Part print with two shaded views. Sizes in mm from the minimum x, y, z corner. Round coordinates to 2 decimals unless told otherwise and drop trailing zeros. Order: outer loops, then holes, each group sorted by start corner. A loop starts at its lowest first (then second) coordinate and runs counter-clockwise, first axis right, second up. Notation, with made-up numbers: (26, -2) - (80, -2) arc R20 cw to (80, 13) - close; hole circle Ø7 at (86.5, 31.5). An arc over 180 degrees is marked (long way). Write item = value, one per line.
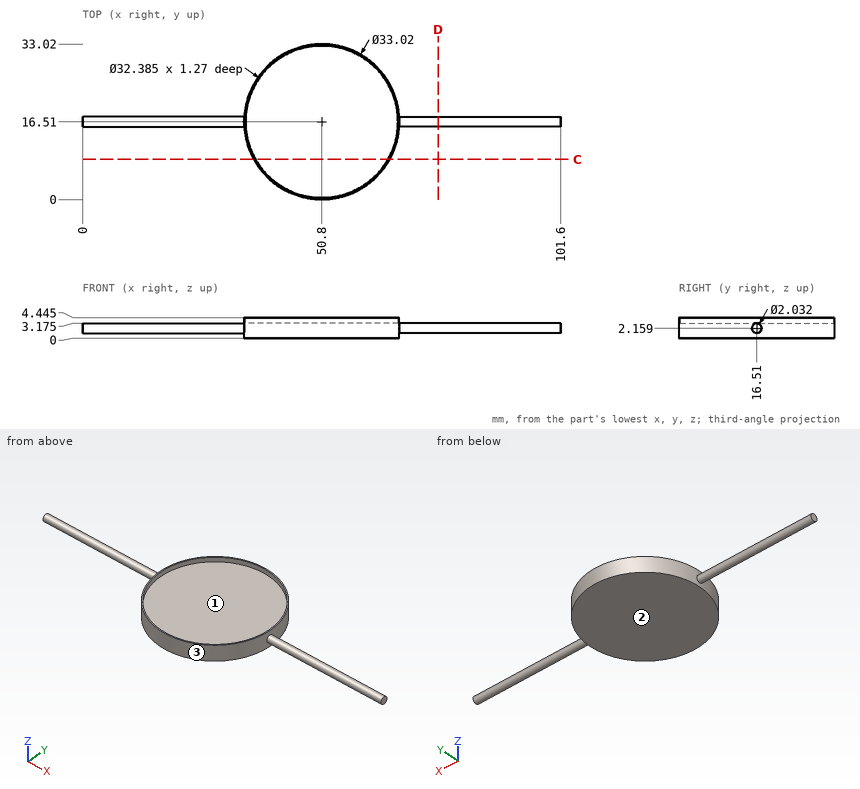
1) Cut at D-D (x = 75.5). Write the cut outline in (y, z).
Conclusion:
outline = circle Ø2.03 at (16.51, 2.16)
2) Flat gauge pins, fed straight in: pin 1 Ø1.5 at (x, z) = (89, 3.5) entering from +Y; pin 2 Ø2 at (x, z) = (78.5, 2.5) entering from +Y; pin 3 Ø10 at (x, y) = (21.5, 12.5) entering from +Z (3 decimals). Where does each tip first touch, or does it go through?
Conclusion:
pin_1 = 17.34
pin_2 = 17.53
pin_3 = 3.175
3) Cut at C-C (y = 8.5). Write the cut outline in (x, z) (3 decimals).
Conclusion:
outline = (36.363, 0) - (65.237, 0) - (65.237, 4.445) - (64.873, 4.445) - (64.873, 3.175) - (36.727, 3.175) - (36.727, 4.445) - (36.363, 4.445) - close
4) Wall check: line 1 along Y through (x, z) = (50.8, 3.75); line 2 along Z through (x, y) = (62.5, 27.5) (3 decimals); line 3 along X through (y, z) = (15, 3.65). Give the ranges that are in metal, low to high.
Conclusion:
line_1 = 0 to 0.32, 32.7 to 33.02
line_2 = 0 to 3.175
line_3 = 34.36 to 34.68, 66.92 to 67.24
5) Mould opens along X. For the marked faces 1, 2 and 3 say: +X half, -X half, draft (parallel to the pull), parting line (faces both ways), or undercut.
Conclusion:
face_1 = undercut
face_2 = draft
face_3 = parting line
